from build123d import *

# Parameters (mm, degrees)
SKETCH1_R              = 1.6
BOSS_EXTRUDE1_DEPTH    = 12.7
SKETCH6_R              = 5.1
CUT_EXTRUDE2_DEPTH     = 84.93709
FILLET1_R              = 5
SKETCH7_R              = 57.15
SKETCH7_R_2            = 44.45
ANALYSIS_SUPPORT_DEPTH = 1


with BuildPart() as part:
    # Sketch1 → Boss-Extrude1 (new body)
    with BuildSketch(Plane.XY):
        with BuildLine():
            Line((54.40471, 17.5), (58.249657, 15))
            ThreePointArc((58.249657, 15), (60.15, 0), (58.249657, -15))
            Line((58.249657, -15), (54.40471, -17.5))
            ThreePointArc((54.40471, -17.5), (0, -57.15), (-54.40471, -17.5))
            Line((-54.40471, -17.5), (-58.249657, -15))
            ThreePointArc((-58.249657, -15), (-60.15, 0), (-58.249657, 15))
            Line((-58.249657, 15), (-54.40471, 17.5))
            ThreePointArc((-54.40471, 17.5), (0, 57.15), (54.40471, 17.5))
        make_face()
        with Locations((0, 53.975)):
            Circle(SKETCH1_R, mode=Mode.SUBTRACT)
        with Locations((46.743721, 26.9875)):
            Circle(SKETCH1_R, mode=Mode.SUBTRACT)
        with Locations((46.743721, -26.9875)):
            Circle(SKETCH1_R, mode=Mode.SUBTRACT)
        with Locations((0, -53.975)):
            Circle(SKETCH1_R, mode=Mode.SUBTRACT)
        with Locations((-46.743721, -26.9875)):
            Circle(SKETCH1_R, mode=Mode.SUBTRACT)
        with Locations((-46.743721, 26.9875)):
            Circle(SKETCH1_R, mode=Mode.SUBTRACT)
    extrude(amount=BOSS_EXTRUDE1_DEPTH)

    # Sketch6 → Cut-Extrude2 (cut, through all)
    with BuildSketch(Plane(origin=(0, 0, 0), x_dir=(-1, 0, 0), z_dir=(0, 0, -1))):
        with Locations((14.551632, 27.5)):
            Circle(SKETCH6_R)
        with Locations((-29.103264, 11)):
            Circle(SKETCH6_R)
        with Locations((-29.103264, -11)):
            Circle(SKETCH6_R)
        with Locations((29.103264, -11)):
            Circle(SKETCH6_R)
        with Locations((29.103264, 11)):
            Circle(SKETCH6_R)
        with Locations((-14.551632, 27.5)):
            Circle(SKETCH6_R)
        with Locations((0, -11)):
            Circle(SKETCH6_R)
        with Locations((-14.551632, -27.5)):
            Circle(SKETCH6_R)
        with Locations((0, 11)):
            Circle(SKETCH6_R)
        with Locations((14.551632, -27.5)):
            Circle(SKETCH6_R)
    extrude(amount=-CUT_EXTRUDE2_DEPTH, mode=Mode.SUBTRACT)

    # Fillet1
    fillet1_edges = [part.edges().sort_by_distance(p)[0] for p in [
        (54.40471, 17.5, 6.35),
        (58.249657, 15, 6.35),
        (58.249657, -15, 6.35),
        (54.40471, -17.5, 6.35),
        (-54.40471, -17.5, 6.35),
        (-58.249657, -15, 6.35),
        (-58.249657, 15, 6.35),
        (-54.40471, 17.5, 6.35),
    ]]
    fillet(fillet1_edges, radius=FILLET1_R)

    # Sketch7 → ANALYSIS-SUPPORT (add)
    with BuildSketch(Plane.XY.offset(12.7)):
        with Locations(Location((0, 0, 0), (0, 0, 160.500332))):
            Circle(SKETCH7_R)
        Circle(SKETCH7_R_2, mode=Mode.SUBTRACT)
    extrude(amount=ANALYSIS_SUPPORT_DEPTH)


solid = part.part
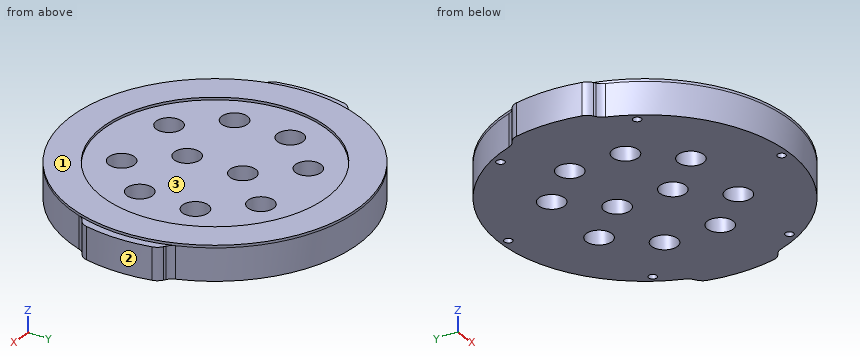
The listing builds one solid part. Answer for the finished solid, in the listing's coordinates (mm). Face numbers are marked on the shaded views. Give positions to 0.01 mm unless a question says otherwise; leave off trailing zeros. Loops run counter-clockwise (first coordinate to the right, second up) from the corner with the lowest first, then second, coordinate; pieces in that order, holes last. Notation, with made-up numbers: (17.5, 17.25) - (50.5, 17.25) arc R19 cw to (50.5, 34.25) - close; hole circle Ø6 at (71.5, 21). An arc over 180 degrees is marked (long way). Answer as a JSON object with one key per item and string values.
1. A cutting plane is placed at D-D (x = 13.5). Write down the section's boundary in (y, z), then the cut area to 3 significant figures.
Determined:
{"outline": "(-55.53, 0) - (-32.49, 0) - (-32.49, 12.7) - (-42.35, 12.7) - (-42.35, 13.7) - (-55.53, 13.7) - close; (-22.51, 0) - (22.51, 0) - (22.51, 12.7) - (-22.51, 12.7) - close; (32.49, 0) - (55.53, 0) - (55.53, 13.7) - (42.35, 13.7) - (42.35, 12.7) - (32.49, 12.7) - close", "area": "1,180 mm²"}
2. A cutting plane is placed at A-A (x = 0). Write down the section's boundary in (y, z) (3 decimals), then the cut area to 3 significant figures.
Determined:
{"outline": "(-57.15, 0) - (-55.575, 0) - (-55.575, 12.7) - (-52.375, 12.7) - (-52.375, 0) - (-16.1, 0) - (-16.1, 12.7) - (-44.45, 12.7) - (-44.45, 13.7) - (-57.15, 13.7) - close; (-5.9, 0) - (5.9, 0) - (5.9, 12.7) - (-5.9, 12.7) - close; (16.1, 0) - (52.375, 0) - (52.375, 12.7) - (55.575, 12.7) - (55.575, 0) - (57.15, 0) - (57.15, 13.7) - (44.45, 13.7) - (44.45, 12.7) - (16.1, 12.7) - close", "area": "1,140 mm²"}
3. Find the intervals of material crossed by L1, parallel to X at y = -29, z = 3; L2, parallel to X at y = -24, z = 10; L3, parallel to Y at x = -14, z = 1.5, in increasing order. Write a range as [from, to].
Determined:
{"L1": "[-49.25, -19.43], [-9.68, 9.68], [19.43, 49.25]", "L2": "[-51.87, -18.26], [-10.84, 10.84], [18.26, 51.87]", "L3": "[-55.41, -32.57], [-22.43, 22.43], [32.57, 55.41]"}
4. For a pull along X with two mould halves and no side action, classify the marked faces 1, 2 and 3 as pulls with the +X half, pulls with the -X half, needs draft (parallel to the pull), parting line crosses it, or undercut.
Determined:
{"face 1": "needs draft", "face 2": "pulls with the +X half", "face 3": "undercut"}
5. A cutting plane is placed at B-B (y = 0). Write down the section's boundary in (x, z), then the cut area to 3 significant figures.
Determined:
{"outline": "(-60.15, 0) - (60.15, 0) - (60.15, 12.7) - (57.15, 12.7) - (57.15, 13.7) - (44.45, 13.7) - (44.45, 12.7) - (-44.45, 12.7) - (-44.45, 13.7) - (-57.15, 13.7) - (-57.15, 12.7) - (-60.15, 12.7) - close", "area": "1,550 mm²"}
6. A cutting plane is placed at C-C (z = 10). Give the number of separate pieces and of enclosed holes in the cut face, then the cut area to 3 significant figures.
Determined:
{"separate pieces": "1", "enclosed holes": "16", "area": "9,590 mm²"}
7. Flat-ended cylindrical pins translate along their axes: pin 1 Ø4 at (x, z) = (-34, 2) entering from +Y; pin 2 Ø8 at (y, z) = (4, 5) entering from +X; pin 3 Ø2 at (y, z) = (-34.5, 2) entering from +X. Find the tip coordinate at first contact, or state that the pin passes through.
Determined:
{"pin 1": "y = 47.35", "pin 2": "x = 60.15", "pin 3": "x = 46.3"}
